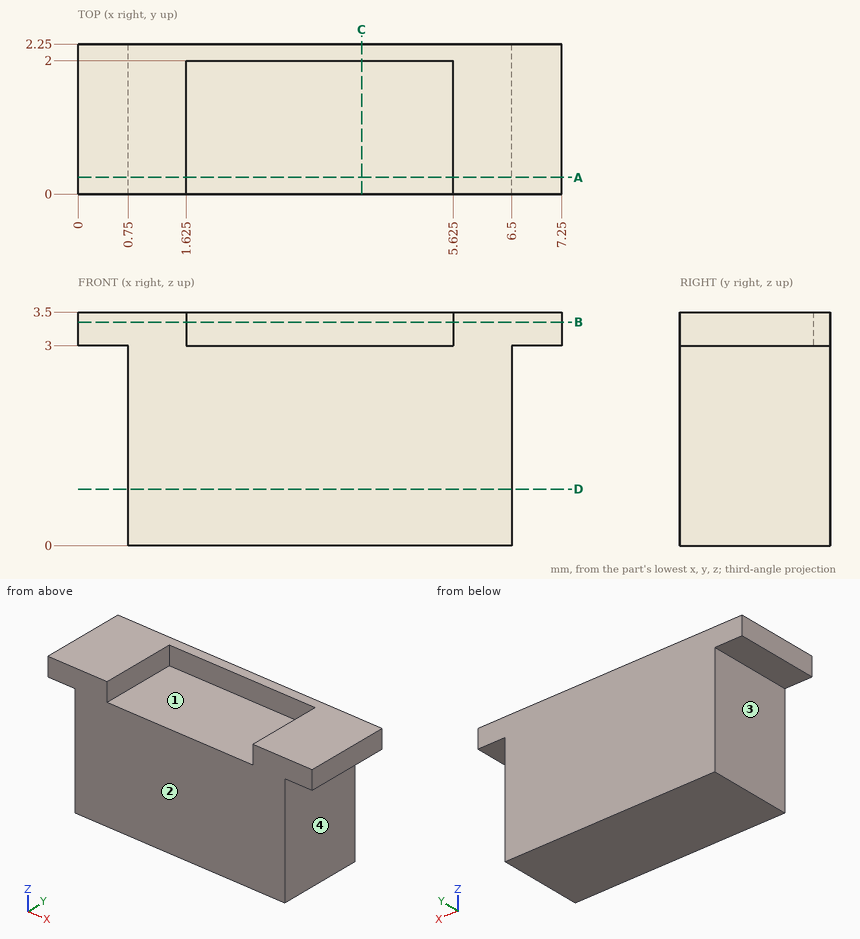
Could you check a few things on this drawing? It's one solid part, dimensions in mm from its lowest x, y, z. Coordinates: 2 decimals unless noted, no trailing zeros. Order: outer loops, then holes, each group sorted by start corner. A loop starts at its lowest first (then second) coordinate and runs counter-clockwise, first axis right, second up.
1) Will these pins go through, and if not, where does the flat tip stop? pin 1 (0.8 mm diameter, centred on x = 7, y = 1, fed in from -Z); pin 2 (0.6 mm diameter, centred on x = 2.5, y = 0.5, fed in from +Z); pin 3 (0.6 mm diameter, centred on x = 4, z = 3, fed in from -Y).
2) We'd pull the mould along X, two halves only. Please class the marked faces 1, 2, 3 and 4: +X half, -X half, draft (parallel to the pull), parting line (faces both ways), or undercut.
3) Imagine slicing it at B-B on z = 3.35. List the corners of the cut face in (x, y) for me (3 decimals).
4) Imagine slicing it at C-C on x = 4.25. List the corners of the cut face in (y, z) for me, and give its area (4 significant figures).
5) I need wall thicknesses on line 1 (X direction, y = 0.25, z = 3.2) (3 decimals); line 2 (Y direction, x = 5, z = 3.2); line 3 (Z direction, x = 3.25, y = 0.25). Which ranges of each line are inside material? Lowest first, please.
6) Imagine slicing it at A-A on y = 0.25. List the corners of the cut face in (x, z) for me (3 decimals).
7) Imagine slicing it at D-D on z = 0.85. List the corners of the cut face in (x, y) for me.
Response values:
1. pin 1: stops at z = 3
1. pin 2: stops at z = 3
1. pin 3: stops at y = 0
2. face 1: undercut
2. face 2: draft
2. face 3: -X half
2. face 4: +X half
3. outline: (0, 0) - (1.625, 0) - (1.625, 2) - (5.625, 2) - (5.625, 0) - (7.25, 0) - (7.25, 2.25) - (0, 2.25) - close
4. outline: (0, 0) - (2.25, 0) - (2.25, 3.5) - (2, 3.5) - (2, 3) - (0, 3) - close
4. area: 6.875 mm2
5. line 1: x = 0 to 1.625, 5.625 to 7.25
5. line 2: y = 2 to 2.25
5. line 3: z = 0 to 3
6. outline: (0, 3) - (0.75, 3) - (0.75, 0) - (6.5, 0) - (6.5, 3) - (7.25, 3) - (7.25, 3.5) - (5.625, 3.5) - (5.625, 3) - (1.625, 3) - (1.625, 3.5) - (0, 3.5) - close
7. outline: (0.75, 0) - (6.5, 0) - (6.5, 2.25) - (0.75, 2.25) - close
